Input: part model. Units: mm. Frame: model coordinates. Face numbers are marked on the shaded views. A direction names the side the tool comes from. Coordinates: 2 decimals unless noted, no trailing zeros. Write each loop counter-clockwise with the first axis right and the second up, starting at its lowest first coordinate (ties: lowest second). Pieces come first, ordered by that corner, then holes. Notation, with made-up numbers: M 2,-14.75 L 16,-14.75 A10 cw 16,0.25 Z; hole C 50.25,-29 d3. An arc over 180 degrees is marked long. Answer as a JSON object with one key per item and string values. Group by question number.
from build123d import *

# Parameters (mm, degrees)
SKETCH2_R               = 88.9
SKETCH2_R_2             = 38.1
BOSS_EXTRUDE1_DEPTH     = 3.175
SKETCH2_4_W             = 101.6
SKETCH2_4_H             = 101.6
SKETCH2_4_W_2           = 95.25
SKETCH2_4_H_2           = 95.25
BOSS_EXTRUDE2_DEPTH     = 266.7
SKETCH3_R               = 88.9
SKETCH3_R_2             = 38.1
BOSS_EXTRUDE3_DEPTH     = 3.175
SKETCH4_W               = 63.5
SKETCH4_H               = 222.25
CUT_EXTRUDE1_DEPTH      = 89.9
CUT_EXTRUDE1_DEPTH_BACK = 89.9
SKETCH5_W               = 63.5
SKETCH5_H               = 222.25
CUT_EXTRUDE2_DEPTH      = 89.9
CUT_EXTRUDE2_DEPTH_BACK = 89.9


with BuildPart() as part:
    # Sketch2 → Boss-Extrude1 (new body)
    with BuildSketch(Plane(origin=(0, 0, 0), x_dir=(1, 0, 0), z_dir=(0, 1, 0))):
        Circle(SKETCH2_R)
        Circle(SKETCH2_R_2, mode=Mode.SUBTRACT)
    extrude(amount=BOSS_EXTRUDE1_DEPTH)

    # Sketch2<4> → Boss-Extrude2 (add)
    with BuildSketch(Plane(origin=(0, 0, 0), x_dir=(1, 0, 0), z_dir=(0, 1, 0))):
        Rectangle(SKETCH2_4_W, SKETCH2_4_H)
        Rectangle(SKETCH2_4_W_2, SKETCH2_4_H_2, mode=Mode.SUBTRACT)
    extrude(amount=BOSS_EXTRUDE2_DEPTH)

    # Sketch3 → Boss-Extrude3 (add)
    with BuildSketch(Plane(origin=(0, 266.7, 0), x_dir=(1, 0, 0), z_dir=(0, 1, 0))):
        Circle(SKETCH3_R)
        Circle(SKETCH3_R_2, mode=Mode.SUBTRACT)
    extrude(amount=-BOSS_EXTRUDE3_DEPTH)

    # Sketch4 → Cut-Extrude1 (cut, two sides)
    with BuildSketch(Plane.XY) as cut_extrude1_sk:
        with Locations((0, 133.35)):
            Rectangle(SKETCH4_W, SKETCH4_H)
    extrude(amount=CUT_EXTRUDE1_DEPTH, mode=Mode.SUBTRACT)
    extrude(cut_extrude1_sk.sketch, amount=-CUT_EXTRUDE1_DEPTH_BACK, mode=Mode.SUBTRACT)

    # Sketch5 → Cut-Extrude2 (cut, two sides)
    with BuildSketch(Plane(origin=(0, 0, 0), x_dir=(0, 0, -1), z_dir=(1, 0, 0))) as cut_extrude2_sk:
        with Locations((0, 133.35)):
            Rectangle(SKETCH5_W, SKETCH5_H)
    extrude(amount=CUT_EXTRUDE2_DEPTH, mode=Mode.SUBTRACT)
    extrude(cut_extrude2_sk.sketch, amount=-CUT_EXTRUDE2_DEPTH_BACK, mode=Mode.SUBTRACT)


solid = part.part
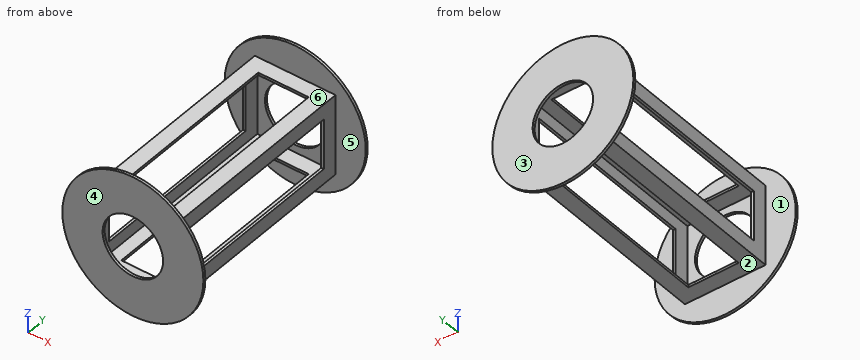
Q1. Section A-A, the plane z = 0. State how many separate pieces and enclosed holes the cut face has, and give its area (3 significant figures).
Q2. Section D-D, the plane z = -62. Return the cut outline in (x, y) (3 decimals), and give its area (3 significant figures).
Q3. Pin query (flat end, axial travel): pin 1 Ø1.6 at (x, z) = (49, -10) entering from -Y; pin 2 Ø2.5 at (y, z) = (98, 49) entering from +X; pin 3 Ø1 at (x, y) = (-49, 86) entering from +Z; pin 4 Ø2 at (y, z) = (199.5, 35) entering from -X. Return the tip coordinate at first contact, or that it passes through.
Q4. Access query for the marked faces 1 and 2. Directions: +Z, -Z, +X, -X, +Y, -Y. A direction counts if a zero-diameter tool reaches every point of the face in a straight line with its end or side. Return the directions, or none.
Q5. Section B-B, the plane y = 101. Return the cut outline in (x, z) (3 decimals), and give its area (3 significant figures).
Q6. Line query: line 1 (X direction, y = 251, z = -28) (3 decimals); line 2 (Y direction, x = 46, z = -2) (3 decimals); line 3 (X direction, y = 1.85, z = 0). Output: solid intervals per line, ascending. Write a range as from..to.
Q7. Draft query along Y for the marked faces 3, 4, 5 and 6. Return one class per face: released by +Y, released by -Y, zero draft, split by the parting line, or undercut.
Filled in:
{
 "1": {"separate pieces": "4", "enclosed holes": "0", "area": "887 mm^2"},
 "2": {"outline": "M -63.712,0 L 63.712,0 L 63.712,3.175 L -63.712,3.175 Z; M -63.712,263.525 L 63.712,263.525 L 63.712,266.7 L -63.712,266.7 Z", "area": "809 mm^2"},
 "3": {"pin 1": "y = 0", "pin 2": "x = 50.8", "pin 3": "z = 50.8", "pin 4": "x = -50.8"},
 "4": {"face 1": "none", "face 2": "-Z, +X, -X"},
 "5": {"outline": "M -50.8,-50.8 L -31.75,-50.8 L -31.75,-47.625 L -47.625,-47.625 L -47.625,-31.75 L -50.8,-31.75 Z; M -50.8,31.75 L -47.625,31.75 L -47.625,47.625 L -31.75,47.625 L -31.75,50.8 L -50.8,50.8 Z; M 31.75,-50.8 L 50.8,-50.8 L 50.8,-31.75 L 47.625,-31.75 L 47.625,-47.625 L 31.75,-47.625 Z; M 31.75,47.625 L 47.625,47.625 L 47.625,31.75 L 50.8,31.75 L 50.8,50.8 L 31.75,50.8 Z", "area": "444 mm^2"},
 "6": {"line 1": "-50.8..-47.625, 47.625..50.8", "line 2": "0..3.175, 263.525..266.7", "line 3": "-88.9..-38.1, 38.1..88.9"},
 "7": {"face 3": "released by +Y", "face 4": "released by -Y", "face 5": "undercut", "face 6": "undercut"}
}
